from build123d import *

# Parameters (mm, degrees)
EXTRUDE_1_DEPTH = 6
CHAMFER_1_SIZE  = 1.5


with BuildPart() as part:
    # 草图1 → 凸台-拉伸1 (new body)
    with BuildSketch(Plane(origin=(0, 0, 0), x_dir=(0, 0, -1), z_dir=(1, 0, 0))):
        Polygon((0, 8.082903769), (7, 4.041451884), (7, -4.041451884), (0, -8.082903769), (-7, -4.041451884), (-7, 4.041451884), align=None)
    extrude(amount=-EXTRUDE_1_DEPTH)

    # 草图3 → 旋转1 (revolve)
    with BuildSketch(Plane.XY, mode=Mode.PRIVATE) as revolve_1_sk:
        Polygon((-6, 6.5), (-7, 6.5), (-7, 4.25), (-9, 4.25), (-9, 5), (-15, 5), (-15, 0), (-6, 0), align=None)
    revolve(revolve_1_sk.sketch.rotate(Axis((10.611885909, 0, 0), (-1, 0, 0)), 90), axis=Axis((10.611885909, 0, 0), (-1, 0, 0)))

    # 草图4 → 切除-旋转1 (revolve, cut)
    with BuildSketch(Plane.XY):
        Polygon((0, -7), (-1.467666471, -9.542072896), (2.047412029, -9.542072896), align=None)
    revolve(axis=Axis((-15, 0, 0), (1, 0, 0)), mode=Mode.SUBTRACT)

    # 倒角1
    chamfer_1_edges = [part.edges().sort_by_distance(p)[0] for p in [
        (-15, 0, 5),
    ]]
    chamfer(chamfer_1_edges, length=CHAMFER_1_SIZE)


solid = part.part
For this review, take the finished solid that the model builds, in its own axes (mm). A direction names the side the tool comes from. Coordinates: 2 decimals unless noted, no trailing zeros. Order: outer loops, then holes, each group sorted by start corner. A loop starts at its lowest first (then second) coordinate and runs counter-clockwise, first axis right, second up. Notation, with made-up numbers: (-28.75, -1.75) - (-10.75, -1.75) arc R18 ccw to (-10.75, 2.25) - close; hole circle Ø3 at (32.25, 87.5). An arc over 180 degrees is marked (long way). Answer as CSV lines item,"result". Start each with the question number.
1) Draft analysis for pull direction X (two halves, no side actions). For faces 1 (the flat face through (-9, 4, -2)), 2 (the cylindrical face through (-11, 0, 5)), 3 (the flat face through (-15, 0, 0)), state which applies: +X half, -X half, draft (parallel to the pull), parting line (faces both ways), or undercut.
2) Add section C-C (x = -13.25). State the section outline as (y, z) points, then the cut area to 3 significant figures.
3) Add section A-A (x = -5). State the section outline as (y, z) points, then the cut area to 3 significant figures.
4) Insertion check: P1, Ø2, axis at x = -6, y = 5.5, coming from the -Z side; P2, Ø3, axis at x = -11.5, z = -5, coming from the -Y side; P3, Ø6, axis at x = -3, z = -5, coming from the +Y side. Each pin has a flat end and moves straight along its axis. Give the tip position at first contact, or say it passes through.
5) To check wall thickness, follow line 1 along X through (y, z) = (-5, 3.25); line 2 along X through (y, z) = (-6.75, 1.75); line 3 along Z through (x, y) = (-6.25, -5.25). State the ranges of each line that lie inside material, in increasing order. Write a range as [from, to].
6) Add section B-B (x = -7.75). State the section outline as (y, z) points, then the cut area to 3 significant figures.
7) Machinability: for faces 4 (the cylindrical face through (-6.507, 3.955, 5.158)), 5 (the flat face through (-3, 0, 7)), 6 (the cylindrical face through (-8.014, -4.214, 0.553)), which of the approach directions +Z, -Z, +X, -X, +Y, -Y give a long, thin tool a straight path to every point of the face, cutting with its end or side? Answer none if there is none.
Result:
1,face 1,"undercut"
1,face 2,"draft"
1,face 3,"-X half"
2,outline,"circle Ø10 at (0, 0)"
2,area,"78.5 mm^2"
3,outline,"(-8.08, 0) - (-4.04, -7) - (4.04, -7) - (8.08, 0) - (4.04, 7) - (-4.04, 7) - close"
3,area,"170 mm^2"
4,P1,"z = -6.21"
4,P2,"y = -3.57"
4,P3,"y = 6.93"
5,line 1,"[-7, 0]"
5,line 2,"[-6, 0]"
5,line 3,"[-3.83, 3.83]"
6,outline,"circle Ø8.5 at (0, 0)"
6,area,"56.7 mm^2"
7,face 4,"-X"
7,face 5,"+Z, +X, -X, +Y, -Y"
7,face 6,"none"
